The listing builds one solid part. Answer for the finished solid, in the listing's coordinates (mm). Coordinates: 2 decimals unless noted, no trailing zeros. Order: outer loops, then holes, each group sorted by start corner. A loop starts at its lowest first (then second) coordinate and runs counter-clockwise, first axis right, second up. Notation, with made-up numbers: (80.25, -33.75) - (89.25, -33.75) arc R23 cw to (89.25, -22.75) - close; hole circle Ø8 at (-22, 34.25). An arc over 180 degrees is marked (long way). Use a Markdown table: item, result. Add a question column.
Item 1: The part is cut by section A-A, the plane x = 6.5. Give the vertices of the cut face in (y, z).
Item 2: A flat-ended cylindrical pin translates along its axis: P1, Ø2.5, axis at x = 7.5, y = 4.69, coming from the +Z side. Find the tip coordinate at first contact, or state that the pin passes through.
Item 3: The mould has two halves that part along Y. Classify faces 1 (the cylindrical face through (6.33, 17.69, 0.01)), 2 (the cylindrical face through (6.47, 5.63, -0.01)), 3 (the flat face through (6.67, -0.86, 0.01)): released by +Y, released by -Y, zero draft, split by the parting line, or undercut.
Item 4: The part is cut by section C-C, the plane y = 10. Give the vertices of the cut face in (x, z).
Item 5: The part is cut by section D-D, the plane x = 11.25. Give the vertices of the cut face in (y, z).
Item 6: The part is cut by section B-B, the plane z = 0. Give the vertices of the cut face in (x, y), then the cut area to 3 significant figures.
Item 7: Find the intervals of material crossed by line 1 along Y through (x, z) = (10, 0.3); line 2 along X through (y, z) = (17.5, 0.05); line 3 along X through (y, z) = (-4.5, -0.15), in increasing order.
from build123d import *

# Parameters (mm, degrees)
SKETCH1_R           = 1.397
BOSS_EXTRUDE1_DEPTH = 0.4445
CUT_EXTRUDE4_DEPTH  = 16.51


with BuildPart() as part:
    # Sketch1 → Boss-Extrude1 (new body, symmetric)
    with BuildSketch(Plane.XY):
        with BuildLine():
            Line((8.875350221, 21.396721542), (9.593451212, 8.117540032))
            ThreePointArc((9.593451212, 8.117540032), (9.965793887, 7.218625297), (10.864708622, 6.846282623))
            ThreePointArc((10.864708622, 6.846282623), (10.617082025, -2.734099475), (11.797183673, -12.24474615))
            ThreePointArc((11.797183673, -12.24474615), (11.337518417, -13.544150853), (10.014382728, -13.158072262))
            ThreePointArc((10.014382728, -13.158072262), (9.129349257, -12.193661404), (8.721848155, -10.949750073))
            Line((8.721848155, -10.949750073), (8.027558013, -2.912032354))
            ThreePointArc((8.027558013, -2.912032354), (7.861230576, -2.018292431), (7.257903508, -1.338268672))
            Line((7.257903508, -1.338268672), (6.065443849, -0.36416915))
            ThreePointArc((6.065443849, -0.36416915), (5.635017487, 0.104064915), (5.461813548, 0.716037454))
            Line((5.461813548, 0.716037454), (5.388890296, 1.679566547))
            ThreePointArc((5.388890296, 1.679566547), (5.241652075, 2.085780608), (4.868329056, 2.303309644))
            Line((4.868329056, 2.303309644), (4.419812025, 2.47021505))
            ThreePointArc((4.419812025, 2.47021505), (4.011456456, 2.79440081), (3.951939413, 3.312385751))
            Line((3.951939413, 3.312385751), (5.241652075, 13.449796826))
            ThreePointArc((5.241652075, 13.449796826), (6.353290153, 17.745713967), (8.875350221, 21.396721542))
        make_face()
        with Locations((7.503950751, 4.690757252)):
            Circle(SKETCH1_R, mode=Mode.SUBTRACT)
    extrude(amount=BOSS_EXTRUDE1_DEPTH, both=True)

    # Sketch2 → Cut-Extrude4 (cut)
    with BuildSketch(Plane(origin=(-1.305559533, 24.142512274, 0), x_dir=(0.998541027, 0.053998306, 0), z_dir=(-0.053998306, 0.998541027, 0))):
        Polygon((10.017788036, 0.4445), (10.017788036, -0.4445), (9.504523646, -0.4445), align=None)
    extrude(amount=-CUT_EXTRUDE4_DEPTH, mode=Mode.SUBTRACT)


solid = part.part
Solution:
| question | item | result |
|---|---|---|
| 1 | outline | (-0.72, -0.44) - (3.72, -0.44) - (3.72, 0.44) - (-0.72, 0.44) - close; (5.66, -0.44) - (18.06, -0.44) - (18.06, 0.44) - (5.66, 0.44) - close |
| 2 | P1 | passes through |
| 3 | face 1 | released by +Y |
| 3 | face 2 | undercut |
| 3 | face 3 | released by -Y |
| 4 | outline | (4.8, -0.44) - (9.49, -0.44) - (8.98, 0.44) - (4.8, 0.44) - close |
| 5 | outline | (-13.58, -0.44) - (-9.12, -0.44) - (-9.12, 0.44) - (-13.58, 0.44) - close |
| 6 | outline | (3.95, 3.31) arc R0.68 ccw to (4.42, 2.47) - (4.87, 2.3) arc R0.63 cw to (5.39, 1.68) - (5.46, 0.72) arc R1.37 ccw to (6.07, -0.36) - (7.26, -1.34) arc R1.7 cw to (8.03, -2.91) - (8.72, -10.95) arc R3.1 ccw to (10.01, -13.16) arc R1 ccw to (11.8, -12.24) arc R64.25 cw to (10.86, 6.85) arc R1.27 cw to (9.59, 8.12) - (9.59, 8.2) - (9.33, 8.18) - (8.63, 21.14) arc R12.7 ccw to (5.24, 13.45) - close; hole circle Ø2.79 at (7.5, 4.69) |
| 6 | area | 121 mm2 |
| 7 | line 1 | y = -13.15 to 7.19 |
| 7 | line 2 | x = 6.24 to 8.8 |
| 7 | line 3 | x = 8.16 to 10.73 |
